Source: three-view drawing plus pictorial views. Frame: mm from the lowest corner of the part. A direction names the side the tool comes from. Give positions to 0.01 mm unless a question says otherwise; leave off trailing zeros. Loops run counter-clockwise (first coordinate to the right, second up) from the corner with the lowest first, then second, coordinate; pieces in that order, holes last. Notation, with made-up numbers: M -38.5,-6 L 15.5,-6 A27 ccw 15.5,11 Z; hole C 48.25,-28 d9. An arc over 180 degrees is marked long. Answer as a JSON object with one key per item and string values. Group by question number.
1) Section query A-A on z = 34.5. Return loops of the section in (x, y).
2) Section query D-D on z = 16. Return loops of the section in (x, y).
3) Access query for the marked faces 1 and 2. Directions: +Z, -Z, +X, -X, +Y, -Y. A direction counts if a zero-diameter tool reaches every point of the face in a straight line with its end or side. Return the directions, or none.
4) First-contact query: P1, Ø10.5, axis at x = 15.5, z = 23, coming from the -Y side. Flat tip, straight axial feed; report the tip coordinate or a pass-through.
5) Ray query, L1, parallel to X at y = 44, z = 30; L2, parallel to X at y = 29, z = 40; L3, parallel to Y at x = 4, z = 23. Return the intervals inside material, ascending.
6) Section query B-B on y = 17.5. Return loops of the section in (x, z).
7) Section query C-C on x = 20. Return loops of the section in (y, z).
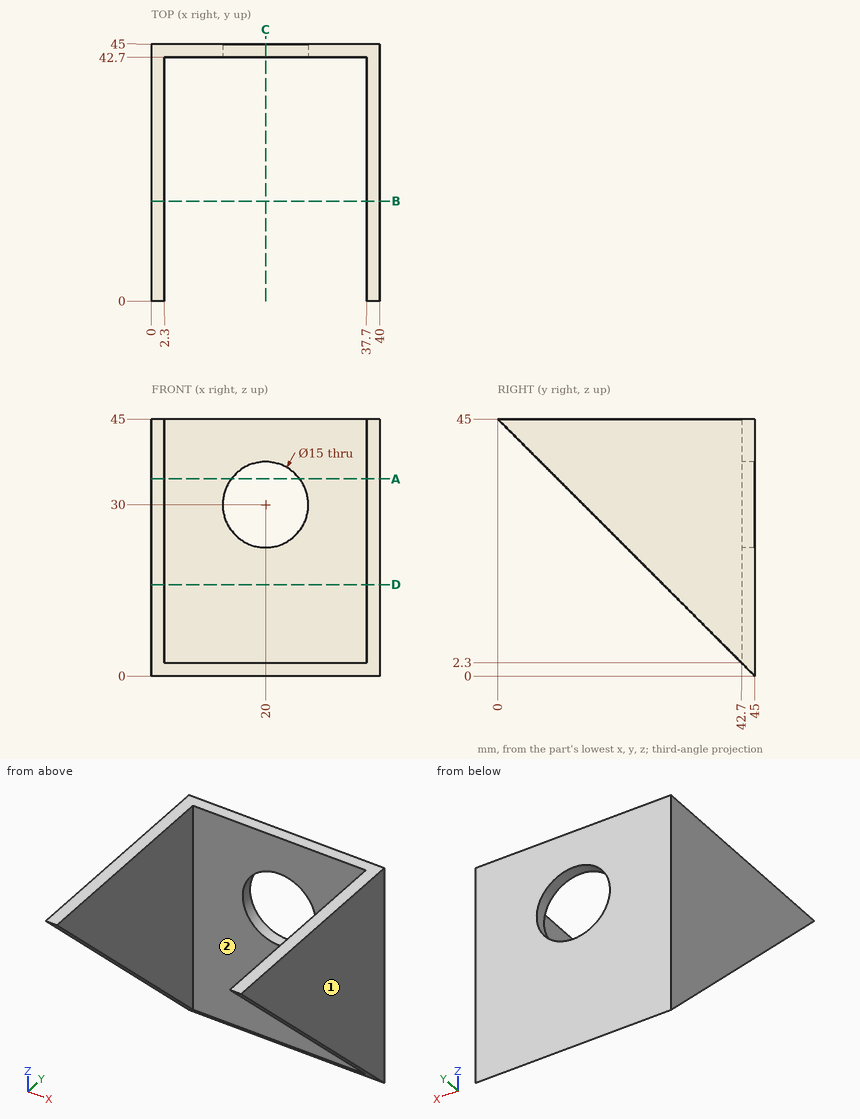
Output:
{
 "1": {"outline": "M 0,10.5 L 2.3,10.5 L 2.3,42.7 L 14,42.7 L 14,45 L 0,45 Z; M 26,42.7 L 37.7,42.7 L 37.7,10.5 L 40,10.5 L 40,45 L 26,45 Z"},
 "2": {"outline": "M 0,29 L 2.3,29 L 2.3,42.7 L 37.7,42.7 L 37.7,29 L 40,29 L 40,45 L 0,45 Z"},
 "3": {"face 1": "+Z, -Z, +X, +Y, -Y", "face 2": "+Z, -Z, -Y"},
 "4": {"P1": "stops at y = 42.7"},
 "5": {"L1": "x = 0 to 12.5, 27.5 to 40", "L2": "x = 0 to 2.3, 37.7 to 40", "L3": "y = 42.7 to 45"},
 "6": {"outline": "M 0,27.5 L 2.3,27.5 L 2.3,45 L 0,45 Z; M 37.7,27.5 L 40,27.5 L 40,45 L 37.7,45 Z"},
 "7": {"outline": "M 42.7,2.3 L 45,0 L 45,22.5 L 42.7,22.5 Z; M 42.7,37.5 L 45,37.5 L 45,45 L 42.7,45 Z"}
}
